Source: CAD feature listing. Evaluate the final solid. Frame: model axes, mm. A direction names the side the tool comes from. Give positions to 0.01 mm unless a question says otherwise; leave off trailing zeros. Order: outer loops, then holes, each group sorted by start corner. A loop starts at its lowest first (then second) coordinate and runs counter-clockwise, first axis right, second up. Notation, with made-up numbers: M -25,-4.5 L -20,-4.5 A36 cw -20,33.5 Z; hole C 83,35.25 d9. An arc over 180 degrees is marked long. Use CSV: the item, a comma, the result in double quotes. Start each with the question number.
1. Reachability of faces 1 (the flat face through (39, 1, 9.3)), 2 (the flat face through (1, 66, 8)), 3 (the flat face through (84, 10, 3.2)) from +Z, -Z, +X, -X, +Y, -Y: full face, straight path, thin tool, end or side. Return the list, or none.
2. Section query A-A, the plane z = 5.25. State how many separate pieces and enclosed holes the cut face has, plus the area to 3 significant figures.
3. Section query D-D, the plane x = 10. Return the cut outline in (y, z), plus the area to 3 significant figures.
4. Pin query (flat end, axial travel): P1, Ø4.5, axis at x = 84.4, y = 89.5, coming from the +Z side; P2, Ø2.5, axis at x = 84.4, y = 10, coming from the +Z side. Return the tip coordinate at first contact, or that it passes through.
5. Section query C-C, the plane y = 71. Return the cut outline in (x, z), plus the area to 3 significant figures.
6. Mould query, pull axis Y, two halves, no side actions, for faces 4 (the flat face through (51, 1, 8)), 5 (the flat face through (47, 99.5, 7)), 6 (the flat face through (3, 49, 8)). Classes: released by +Y, released by -Y, zero draft, split by the parting line, or undercut.
7. Section query B-B, the plane x = 36. Return the cut outline in (y, z).
8. Line query: line 1 along Y through (x, z) = (10, 7.75); line 2 along Y through (x, z) = (9.5, 4); line 3 along X through (y, z) = (54.5, 11.75). Output: solid intervals per line, ascending. Write a range as [from, to].
from build123d import *

# Parameters (mm, degrees)
SKETCH_W        = 94.4
SKETCH_H        = 99.5
PAD_DEPTH       = 13.2
SKETCH001_W     = 88.4
SKETCH001_H     = 93.5
POCKET_DEPTH    = 10
SKETCH002_R     = 3.5
SKETCH002_R_2   = 1.4
PAD001_DEPTH    = 8.5
SKETCH003_W     = 24
SKETCH003_H     = 2.3
POCKET001_DEPTH = 3
SKETCH004_W     = 24
SKETCH004_H     = 5
POCKET002_DEPTH = 3
FILLET_R        = 1.5


with BuildPart() as part:
    # Sketch → Pad (new body)
    with BuildSketch(Plane.XY):
        with Locations((47.2, 49.75)):
            Rectangle(SKETCH_W, SKETCH_H)
    extrude(amount=PAD_DEPTH)

    # Sketch001 (on Face6 of Pad) → Pocket (cut)
    with BuildSketch(Plane.XY.offset(13.2)):
        with Locations((47.2, 49.75)):
            Rectangle(SKETCH001_W, SKETCH001_H)
    extrude(amount=-POCKET_DEPTH, mode=Mode.SUBTRACT)

    # Sketch002 (on Face11 of Pocket) → Pad001 (join)
    with BuildSketch(Plane.XY.offset(3.2)):
        with Locations((84.4, 89.5)):
            Circle(SKETCH002_R)
        with Locations((84.4, 89.5)):
            Circle(SKETCH002_R_2, mode=Mode.SUBTRACT)
        with Locations((10, 89.5)):
            Circle(SKETCH002_R)
        with Locations((10, 89.5)):
            Circle(SKETCH002_R_2, mode=Mode.SUBTRACT)
        with Locations((10, 10)):
            Circle(SKETCH002_R)
        with Locations((10, 10)):
            Circle(SKETCH002_R_2, mode=Mode.SUBTRACT)
        with Locations((84.4, 10)):
            Circle(SKETCH002_R)
        with Locations((84.4, 10)):
            Circle(SKETCH002_R_2, mode=Mode.SUBTRACT)
    extrude(amount=PAD001_DEPTH)

    # Sketch003 (on Face1 of Pad001) → Pocket001 (cut)
    with BuildSketch(Plane.XZ):
        with Locations((39, 8.15)):
            Rectangle(SKETCH003_W, SKETCH003_H)
    extrude(amount=-POCKET001_DEPTH, mode=Mode.SUBTRACT)

    # Sketch004 (on Face2 of Pocket001) → Pocket002 (cut)
    with BuildSketch(Plane(origin=(0, 0, 0), x_dir=(0, -1, 0), z_dir=(-1, 0, 0))):
        with Locations((-65.5, 5.5)):
            Rectangle(SKETCH004_W, SKETCH004_H)
    extrude(amount=-POCKET002_DEPTH, mode=Mode.SUBTRACT)

    # Fillet
    fillet_edges = [part.edges().sort_by_distance(p)[0] for p in [
        (47.2, 0, 0),
        (94.4, 49.75, 0),
        (47.2, 99.5, 0),
        (0, 49.75, 0),
        (94.4, 0, 6.6),
        (0, 0, 6.6),
        (94.4, 99.5, 6.6),
        (0, 99.5, 6.6),
    ]]
    fillet(fillet_edges, radius=FILLET_R)


solid = part.part
Result set:
1,face 1,"-Y"
1,face 2,"-X"
1,face 3,"+Z"
2,separate pieces,"5"
2,enclosed holes,"4"
2,area,"1,180 mm2"
3,outline,"M 0,1.5 A1.5 ccw 1.5,0 L 98,0 A1.5 ccw 99.5,1.5 L 99.5,13.2 L 96.5,13.2 L 96.5,3.2 L 93,3.2 L 93,11.7 L 90.9,11.7 L 90.9,3.2 L 88.1,3.2 L 88.1,11.7 L 86,11.7 L 86,3.2 L 13.5,3.2 L 13.5,11.7 L 11.4,11.7 L 11.4,3.2 L 8.6,3.2 L 8.6,11.7 L 6.5,11.7 L 6.5,3.2 L 3,3.2 L 3,13.2 L 0,13.2 Z"
3,area,"449 mm2"
4,P1,"z = 11.7"
4,P2,"z = 3.2"
5,outline,"M 0,1.5 A1.5 ccw 1.5,0 L 92.9,0 A1.5 ccw 94.4,1.5 L 94.4,13.2 L 91.4,13.2 L 91.4,3.2 L 3,3.2 L 3,3 L 0,3 Z; M 0,8 L 3,8 L 3,13.2 L 0,13.2 Z"
5,area,"346 mm2"
6,face 4,"zero draft"
6,face 5,"released by +Y"
6,face 6,"undercut"
7,outline,"M 0,1.5 A1.5 ccw 1.5,0 L 98,0 A1.5 ccw 99.5,1.5 L 99.5,13.2 L 96.5,13.2 L 96.5,3.2 L 3,3.2 L 3,7 L 0,7 Z; M 0,9.3 L 3,9.3 L 3,13.2 L 0,13.2 Z"
8,line 1,"[0, 3], [6.5, 8.6], [11.4, 13.5], [86, 88.1], [90.9, 93], [96.5, 99.5]"
8,line 2,"[0, 3], [6.54, 8.69], [11.31, 13.46], [86.04, 88.19], [90.81, 92.96], [96.5, 99.5]"
8,line 3,"[0, 3], [91.4, 94.4]"
